```python
from build123d import *

# Parameters (mm, degrees)
RESSALTO_EXTRUS_O3_DEPTH = 25
ESBO_O6_W                = 4
ESBO_O6_H                = 16
RESSALTO_EXTRUS_O6_DEPTH = 24
ESBO_O7_R                = 2
CORTE_EXTRUS_O3_DEPTH    = 43


with BuildPart() as part:
    # Esboço1 → Ressalto-extrusão3 (new body)
    with BuildSketch(Plane.XY):
        Polygon((-3.8, 33.5), (-5.7, 33.5), (-3.940587347, 30.5), (3.940587347, 30.5), (5.7, 33.5), (3.8, 33.5), (3.8, 36.5), (11, 36.5), (11, 29.3), (8, 29.3), (8, 31.2), (5, 29.440587347), (5, 21.559412653), (8, 19.8), (8, 21.7), (11, 21.7), (11, 14.5), (3.8, 14.5), (3.8, 17.5), (5.7, 17.5), (3.940587347, 20.5), (-3.940587347, 20.5), (-5.7, 17.5), (-3.8, 17.5), (-3.8, 14.5), (-11.2, 14.5), (-11.7, 14.5), (-11.7, 10.5), (11.7, 10.5), (15, 10.5), (15, 37.2), (15, 40.5), (-11.7, 40.5), (-11.7, 36.5), (-3.8, 36.5), align=None)
    extrude(amount=RESSALTO_EXTRUS_O3_DEPTH)

    # Esboço6 → Ressalto-extrusão6 (add)
    with BuildSketch(Plane.XY):
        with Locations((13, 44.5)):
            Rectangle(ESBO_O6_W, ESBO_O6_H)
        with Locations((13, 6.5)):
            Rectangle(ESBO_O6_W, ESBO_O6_H)
    extrude(amount=RESSALTO_EXTRUS_O6_DEPTH)

    # Esboço7 → Corte-extrusão3 (cut)
    with BuildSketch(Plane(origin=(0, 0, 0), x_dir=(0, 0, -1), z_dir=(1, 0, 0))):
        with Locations((-12, 46.5)):
            Circle(ESBO_O7_R)
        with Locations((-12, 4.5)):
            Circle(ESBO_O7_R)
    extrude(amount=CORTE_EXTRUS_O3_DEPTH, mode=Mode.SUBTRACT)


solid = part.part
```
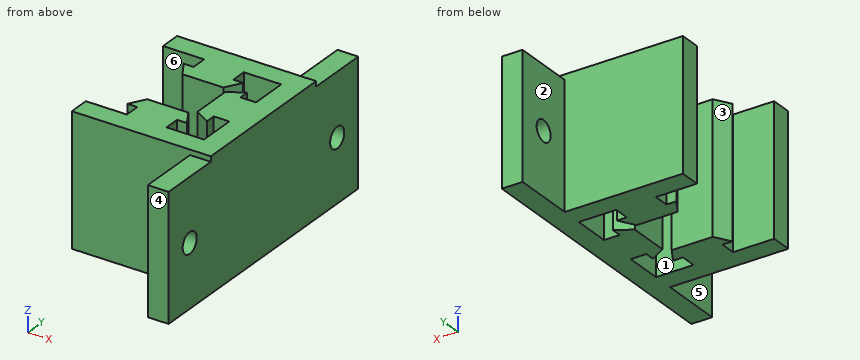
Input: part model. Units: mm. Frame: model coordinates. Face numbers are marked on the shaded views. A direction names the side the tool comes from. Coordinates: 2 decimals unless noted, no trailing zeros. Write each loop counter-clockwise with the first axis right and the second up, starting at its lowest first coordinate (ties: lowest second). Pieces come first, ordered by that corner, then holes.
1) Section D-D on y = 24. Output: boundary loops of the cut face in (x, z).
2) Section C-C on z = 12. State how many separate pieces and enclosed holes the cut face has, and give its area (3 significant figures).
3) Section B-B on x = 6.5. Output: boundary loops of the cut face in (y, z), and give its area (3 significant figures).
4) Section A-A on y = 46.5. Output: boundary loops of the cut face in (x, z), and give its area (3 significant figures).
5) Pin query (flat end, axial travel): pin 1 Ø2.5 at (y, z) = (46.5, 12) entering from -X; pin 2 Ø1.5 at (y, z) = (16, 16.5) entering from -X; pin 3 Ø1.5 at (x, z) = (-5, 12) entering from +Y; pin 4 Ø8 at (y, z) = (21, 5.5) entering from -X. Return the tip coordinate at first contact, or that it passes through.
6) Set-up query: the marked faces 1, 2 and 3. Return all of +Z, -Z, +X, -X, +Y, -Y with unobstructed straight access to the full face (end or side cutting, diameter ignored); none if empty.
7) Material intervals for line 1 along Y through (x, z) = (13.45, 12); line 2 along Y through (x, z) = (-6.25, 12.75); line 3 along Z through (x, y) = (13.15, 4.5), sorted ascending.
8) Mould query, pull axis Y, two halves, no side actions, for the marked faces 4, 5 and 6. Classes: pulls with the +Y half, pulls with the -Y half, needs draft (parallel to the pull), parting line crosses it, or undercut.
Check result:
1. outline: (5, 0) - (15, 0) - (15, 25) - (5, 25) - close
2. separate pieces: 3
2. enclosed holes: 0
2. area: 521 mm2
3. outline: (10.5, 0) - (14.5, 0) - (14.5, 25) - (10.5, 25) - close; (20.68, 0) - (30.32, 0) - (30.32, 25) - (20.68, 25) - close; (36.5, 0) - (40.5, 0) - (40.5, 25) - (36.5, 25) - close
3. area: 441 mm2
4. outline: (11, 0) - (15, 0) - (15, 10) - (11, 10) - close; (11, 14) - (15, 14) - (15, 24) - (11, 24) - close
4. area: 80.0 mm2
5. pin 1: passes through
5. pin 2: stops at x = -3.8
5. pin 3: stops at y = 40.5
5. pin 4: stops at x = -5.7
6. face 1: +Z, -Z
6. face 2: +Z, -Z, -X, +Y
6. face 3: +Z, -Z, -X
7. line 1: y = -1.5 to 2.5, 6.5 to 44.5, 48.5 to 52.5
7. line 2: y = 10.5 to 14.5, 36.5 to 40.5
7. line 3: z = 0 to 10, 14 to 24
8. face 4: pulls with the -Y half
8. face 5: needs draft
8. face 6: undercut
